CAD build for the part. Positions are in the model's coordinates, mm. Coordinates: 2 decimals unless noted, no trailing zeros. Write each loop counter-clockwise with the first axis right and the second up, starting at its lowest first coordinate (ties: lowest second). Pieces come first, ordered by that corner, then holes.
```python
from build123d import *

# Parameters (mm, degrees)
SKETCH1_R           = 190
SKETCH1_R_2         = 2
BOSS_EXTRUDE1_DEPTH = 3.125
SKETCH2_R           = 2
CUT_EXTRUDE2_DEPTH  = 3.125
SKETCH3_R           = 20
CUT_EXTRUDE3_DEPTH  = 3.125


with BuildPart() as part:
    # Sketch1 → Boss-Extrude1 (new body)
    with BuildSketch(Plane(origin=(0, 0, 0), x_dir=(1, 0, 0), z_dir=(0, 1, 0))):
        with Locations(Location((0, 0, 0), (0, 0, 270))):
            Circle(SKETCH1_R)
        with Locations(Location((0, -170, 0), (0, 0, 270))):
            Circle(SKETCH1_R_2, mode=Mode.SUBTRACT)
        with Locations(Location((-170, 0, 0), (0, 0, 270))):
            Circle(SKETCH1_R_2, mode=Mode.SUBTRACT)
        with Locations(Location((0, 170, 0), (0, 0, 270))):
            Circle(SKETCH1_R_2, mode=Mode.SUBTRACT)
        with Locations(Location((170, 0, 0), (0, 0, 270))):
            Circle(SKETCH1_R_2, mode=Mode.SUBTRACT)
        with Locations(Location((-141.715728753, 28.284271247, 0), (0, 0, 270))):
            Circle(SKETCH1_R_2, mode=Mode.SUBTRACT)
        with Locations(Location((-113.431457505, 56.568542495, 0), (0, 0, 270))):
            Circle(SKETCH1_R_2, mode=Mode.SUBTRACT)
        with Locations(Location((-85.147186258, 84.852813742, 0), (0, 0, 270))):
            Circle(SKETCH1_R_2, mode=Mode.SUBTRACT)
        with Locations(Location((-56.86291501, 113.13708499, 0), (0, 0, 270))):
            Circle(SKETCH1_R_2, mode=Mode.SUBTRACT)
        with Locations(Location((-28.578643763, 141.421356237, 0), (0, 0, 270))):
            Circle(SKETCH1_R_2, mode=Mode.SUBTRACT)
        with Locations(Location((-141.715728753, -28.284271247, 0), (0, 0, 270))):
            Circle(SKETCH1_R_2, mode=Mode.SUBTRACT)
        with Locations(Location((28.284271247, 141.715728753, 0), (0, 0, 270))):
            Circle(SKETCH1_R_2, mode=Mode.SUBTRACT)
        with Locations(Location((-113.431457505, -56.568542495, 0), (0, 0, 270))):
            Circle(SKETCH1_R_2, mode=Mode.SUBTRACT)
        with Locations(Location((56.568542495, 113.431457505, 0), (0, 0, 270))):
            Circle(SKETCH1_R_2, mode=Mode.SUBTRACT)
        with Locations(Location((-85.147186258, -84.852813742, 0), (0, 0, 270))):
            Circle(SKETCH1_R_2, mode=Mode.SUBTRACT)
        with Locations(Location((84.852813742, 85.147186258, 0), (0, 0, 270))):
            Circle(SKETCH1_R_2, mode=Mode.SUBTRACT)
        with Locations(Location((-56.86291501, -113.13708499, 0), (0, 0, 270))):
            Circle(SKETCH1_R_2, mode=Mode.SUBTRACT)
        with Locations(Location((113.13708499, 56.86291501, 0), (0, 0, 270))):
            Circle(SKETCH1_R_2, mode=Mode.SUBTRACT)
        with Locations(Location((-28.578643763, -141.421356237, 0), (0, 0, 270))):
            Circle(SKETCH1_R_2, mode=Mode.SUBTRACT)
        with Locations(Location((141.421356237, 28.578643763, 0), (0, 0, 270))):
            Circle(SKETCH1_R_2, mode=Mode.SUBTRACT)
        with Locations(Location((28.284271247, -141.715728753, 0), (0, 0, 270))):
            Circle(SKETCH1_R_2, mode=Mode.SUBTRACT)
        with Locations(Location((56.568542495, -113.431457505, 0), (0, 0, 270))):
            Circle(SKETCH1_R_2, mode=Mode.SUBTRACT)
        with Locations(Location((84.852813742, -85.147186258, 0), (0, 0, 270))):
            Circle(SKETCH1_R_2, mode=Mode.SUBTRACT)
        with Locations(Location((113.13708499, -56.86291501, 0), (0, 0, 270))):
            Circle(SKETCH1_R_2, mode=Mode.SUBTRACT)
        with Locations(Location((141.421356237, -28.578643763, 0), (0, 0, 270))):
            Circle(SKETCH1_R_2, mode=Mode.SUBTRACT)
    extrude(amount=BOSS_EXTRUDE1_DEPTH)

    # Sketch2 → Cut-Extrude2 (cut)
    with BuildSketch(Plane(origin=(0, 3.125, 0), x_dir=(1, 0, 0), z_dir=(0, 1, 0))):
        with Locations(Location((-60, 0, 0), (0, 0, 270))):
            Circle(SKETCH2_R)
        with Locations(Location((0, 60, 0), (0, 0, 270))):
            Circle(SKETCH2_R)
        with Locations(Location((60, 0, 0), (0, 0, 270))):
            Circle(SKETCH2_R)
        with Locations(Location((0, -60, 0), (0, 0, 270))):
            Circle(SKETCH2_R)
    extrude(amount=-CUT_EXTRUDE2_DEPTH, mode=Mode.SUBTRACT)

    # Sketch3 → Cut-Extrude3 (cut)
    with BuildSketch(Plane(origin=(0, 3.125, 0), x_dir=(1, 0, 0), z_dir=(0, 1, 0))):
        with Locations(Location((-114.941299582, 0, 0), (0, 0, 270))):
            Circle(SKETCH3_R)
        with Locations(Location((0, 114.941299582, 0), (0, 0, 270))):
            Circle(SKETCH3_R)
        with Locations(Location((114.941299582, 0, 0), (0, 0, 270))):
            Circle(SKETCH3_R)
        with Locations(Location((0, -114.941299582, 0), (0, 0, 270))):
            Circle(SKETCH3_R)
    extrude(amount=-CUT_EXTRUDE3_DEPTH, mode=Mode.SUBTRACT)


solid = part.part
```
Item 1: Flat gauge pin, fed straight in: pin 1 Ø1.5 at (x, y) = (22, 1.5) entering from +Z. Where does the tip first touch, or does it go through?
Item 2: Saw through at B-B, the plane z = -160. Write the cut outline in (x, y) (1 decimal), and give its area (3 significant figures).
Item 3: Two-plate mould, pull along X, no slides. Class faces 1 (the cylindrical face through (95.417, 1.584, -4.336)), 2 (the flat face through (3, 3.125, -3)), 3 (the cylindrical face through (-185.48, 1.54, -41.19)): +X half, -X half, draft (parallel to the pull), parting line (faces both ways), or undercut.
Item 4: Saw through at A-A, the plane y = 1.15. State how many separate pieces and enclosed holes the cut face has, and give its area (3 significant figures).
Item 5: Wall check: line 1 along Z through (x, y) = (57.5, 1.95); line 2 along X through (y, z) = (1.2, 8); line 3 along Z through (x, y) = (130, 1.1). Give the ranges that are in metal, low to high.
Item 6: Saw through at C-C, the plane x = 68. Write the cut outline in (y, z) (3 decimals).
Working result:
1. pin 1: stops at z = 188.81
2. outline: (-102.5, 0) - (102.5, 0) - (102.5, 3.1) - (-102.5, 3.1) - close
2. area: 640 mm2
3. face 1: undercut
3. face 2: draft
3. face 3: parting line
4. separate pieces: 1
4. enclosed holes: 32
4. area: 108,000 mm2
5. line 1: z = -181.09 to -115.2, -111.66 to 111.66, 115.2 to 181.09
5. line 2: x = -189.83 to -133.27, -96.61 to 96.61, 133.27 to 189.83
5. line 3: z = -138.56 to -13.16, 13.16 to 138.56
6. outline: (0, -177.415) - (3.125, -177.415) - (3.125, 177.415) - (0, 177.415) - close
